Part print with two shaded views. Sizes in mm from the minimum x, y, z corner. A direction names the side the tool comes from. Round coordinates to 2 decimals unless told otherwise and drop trailing zeros. Loops run counter-clockwise (first coordinate to the right, second up) from the corner with the lowest first, then second, coordinate; pieces in that order, holes last.
(1) Tool access for the marked faces 1, 2 and 3: list every direction of +Z, -Z, +X, -X, +Y, -Y with a clear straight run to the whole face (end or side of a thin tool).
(2) Flat gauge pins, fed straight in: pin 1 (3 mm diameter, centred on x = 7.5, y = 10.5, fed in from -Z); pin 2 (3 mm diameter, centred on x = 13.5, y = 1.5, fed in from -Z); pin 3 (3.5 mm diameter, centred on y = 8, z = 7.5, fed in from +X). Where does each tip first touch, or does it go through?
(3) Probe probe 1 along Z at (x, y) = (7.5, 7); probe 2 along Y at (x, z) = (10, 12.5). List the from-to ranges inside material, lowest first.
(4) Mould opens along X. For the marked faces 4, 5 and 6 say: +X half, -X half, draft (parallel to the pull), parting line (faces both ways), or undercut.
(5) Cut at D-D on y = 15. List the corners of the cut face in (x, z), then the cut area to 3 significant figures.
(6) Cut at B-B on x = 7.5. List the corners of the cut face in (y, z).
(7) Cut at A-A on z = 1.5. List the corners of the cut face in (x, y).
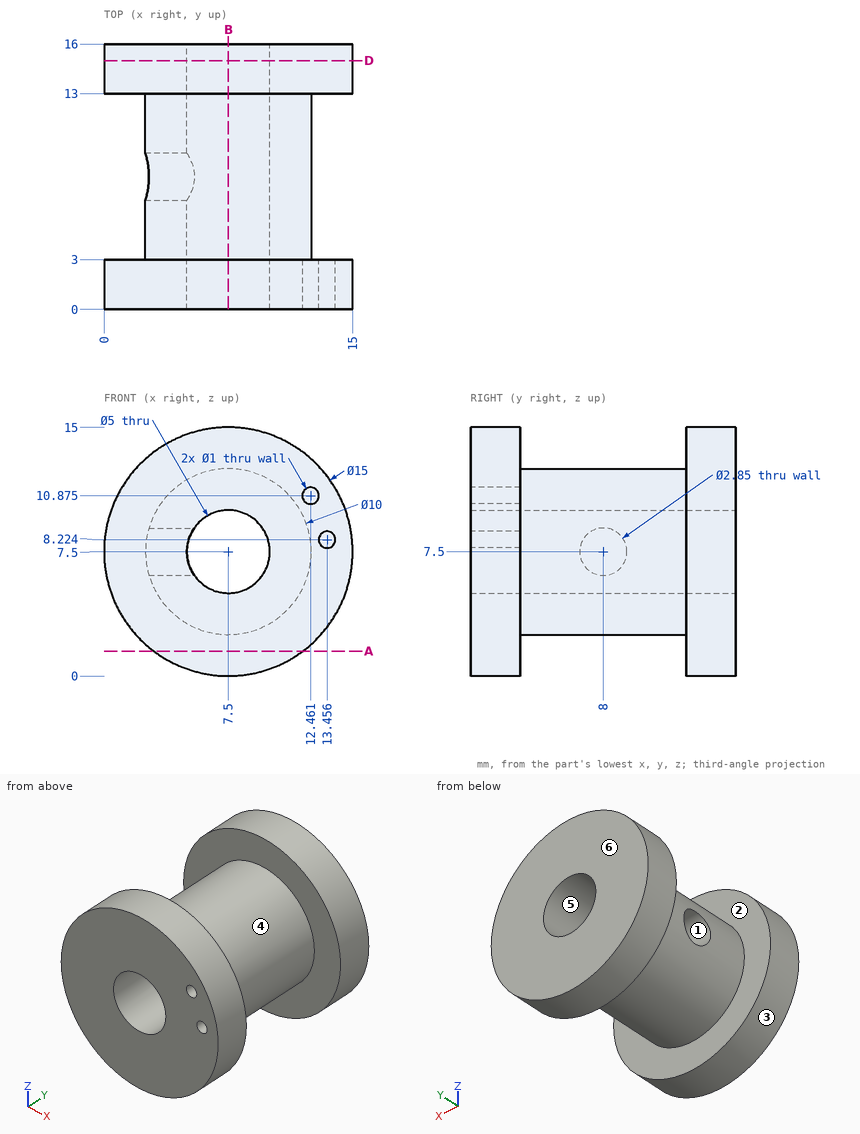
Final values:
1. face 1: -X
1. face 2: none
1. face 3: +Y, -Y
2. pin 1: stops at z = 2.5
2. pin 2: stops at z = 1.5
2. pin 3: stops at x = 12.5
3. probe 1: z = 2.5 to 5, 10 to 12.5
3. probe 2: y = 0 to 3, 13 to 16
4. face 4: parting line
4. face 5: undercut
4. face 6: draft
5. outline: circle Ø15 at (7.5, 7.5); hole circle Ø5 at (7.5, 7.5)
5. area: 157 mm2
6. outline: (0, 0) - (3, 0) - (3, 2.5) - (13, 2.5) - (13, 0) - (16, 0) - (16, 5) - (0, 5) - close; (0, 10) - (16, 10) - (16, 15) - (13, 15) - (13, 12.5) - (3, 12.5) - (3, 15) - (0, 15) - close
7. outline: (3, 0) - (12, 0) - (12, 3) - (3, 3) - close; (3, 13) - (12, 13) - (12, 16) - (3, 16) - close
